Autodesk Inventor part; units mm, degrees
ref_plane "Work Plane1" through (29, 0, 0) normal (0, -1, 0) x (1, 0, 0)
ref_plane "YZ Plane" through (0, 0, 0) normal (1, 0, 0) x (0, 1, 0)
ref_plane "XZ Plane" through (0, 0, 0) normal (0, 1, 0) x (-1, 0, 0)
sketch "Sketch1" plane through (0, 0, 0) normal (0, 0, 1) x (1, 0, 0)
  line L0 (-0.0847, 0) -> (15.875, 0)
  line L1 (15.875, 0) -> (15.875, 2.0828)
  line L2 (15.875, 2.0828) -> (1.5902, 2.0828)
  line L3 (1.5902, 2.0828) -> (0.0001, 2.0828)
  line L4 (0.0001, 2.0828) -> (0, 2.0828)
  line L5 (0, 2.0828) -> (0, 3.9624)
  line L6 (0, 3.9624) -> (-2.2098, 3.9624)
  line L7 (-2.2098, 3.9624) -> (-2.2098, 1.3931)
  line L8 (-2.2098, 1.3931) -> (-0.889, 1.3931)
  line L9 (-0.889, 1.3931) -> (-0.0847, 0)
  line L10 (-21, 0) -> (56, 0)
  line L11 (0, -1.6) -> (0, 9.6)
  line L12 (1.5902, 2.0828) -> (0, 2.0828) construction
  dimension "d1" = 14.2848
  dimension "d2" = 1.5901
  dimension "d3" = 2.2098
  dimension "d4" = 1.3208
  dimension "d5" = 60
  dimension "d6" = 4.1656
  dimension "d7" = 4.1656
  dimension "d8" = 2.7863
  dimension "d9" = 7.9248
  dimension "d26" = 15.875
revolve "Body" add sketch "Sketch1" angle 360 about axis through (-0.0847, 0, 0) along (1, 0, 0)
sketch "Sketch2" plane through (-2.2098, 0, 0) normal (-1, 0, 0) x (0, 0, 1)
  circle A0 centre (0, 0) radius 1.3931
  line L0 (0, -6.4663) -> (0, 6.4663)
  line L1 (-6.4663, 0) -> (6.4663, 0)
  line L2 (1.3931, 0) -> (0.6966, -1.2065)
  line L3 (0.6966, -1.2065) -> (-0.6966, -1.2065)
  line L4 (-0.6966, -1.2065) -> (-1.3931, 0)
  line L5 (-1.3931, 0) -> (-0.6966, 1.2065)
  line L6 (-0.6966, 1.2065) -> (0.6966, 1.2065)
  line L7 (0.6966, 1.2065) -> (1.3931, 0)
extrude "Slot" add sketch "Sketch2" against normal up to next contours L7 A0 | A0 L2 | L6 L0 A0 | A0 L0 L3 | L0 L6 A0 | A0 L3 L0 | L4 A0 | A0 L5
fillet "Fillet1" radius 1.8288 1 edges at (-2.2098, -3.9624, 0)
thread "Thread"
chamfer "Chamfer1" distance 0.4204 distance2 0.4204 1 edges at (15.875, -2.0828, 0) measured on face at (15.875, -0.1898, 0.4203)
ref_plane "Work Plane1" through (29, 0, 0) normal (0, -1, 0) x (1, 0, 0)
fillet "Fillet2" radius 0.1 1 edges at (0.0001, -2.0828, 0)
equation "\"d1\" = GEL"
equation "\"d3\" = KOH"
equation "\"d4\" = INTI"
equation "\"d6\" = GD"
equation "\"d7\" = BDM"
equation "\"d8\" = 1.1547 * SW"
equation "\"d9\" = KOD"
equation "\"d26\" = NLG"
equation "\"d30\" = R"
equation "\"d17\" = RR"
equation "\"d13\" = GEL"
equation "\"d15\" = -0.5 * SPD + 0.5 * GD"
equation "\"d16\" = GUL"
equation "\"GD\" = NND"
equation "\"NLG\" = 15.875"
equation "\"GEL\" = 14.28476"
equation "\"KOD\" = 7.9248"
equation "\"KOH\" = 2.2098"
equation "\"INTI\" = 1.3208"
equation "\"GAL\" = 1.59004"
equation "\"GUL\" = 0.42037"
equation "\"BDM\" = NND"
equation "\"SW\" = 2.413"
equation "\"RR\" = 1.8288"
equation "\"SPD\" = 3.32486"
equation "\"R\" = 0.1"
equation "\"TOA\" = 30deg"
equation "\"GD1\" = SPD"
equation "\"THREADDIA\" = 4.1656"
equation "\"KOH1\" = 0.381"
equation "\"NND\" = 4.1656"
equation "\"E0\" = 2.78714"
properties part number "ANSI B18.3 - No. 8-36 - 5/8" material "Steel, Mild"
Build history of the part. All positions in model axes, mm. A direction names the side the tool comes from. Round coordinates to 2 decimals unless told otherwise and drop trailing zeros. Write each loop counter-clockwise with the first axis right and the second up, starting at its lowest first coordinate (ties: lowest second). Pieces come first, ordered by that corner, then holes.
1) Pin check, flat tips, straight feed: pin 1 (1.5 mm diameter, centred on y = 2, z = 1, fed in from -X); pin 2 (1 mm diameter, centred on x = 2, y = 1, fed in from -Z); pin 3 (2 mm diameter, centred on x = 12.5, z = 1.5, fed in from -Y); pin 4 (2 mm diameter, centred on x = 2, y = -1.5, fed in from +Z). Stop position of each tip, or through.
2) Mould opens along Z. For faces 1 (the conical face through (-0.14, -0.02, 0.09)), 2 (the flat face through (-2.21, -1, 1)), 3 (the cylindrical face through (7.67, 1.987, -0.626)) say: +Z half, -Z half, draft (parallel to the pull), parting line (faces both ways), or undercut.
3) Band-saw the part on A-A, the plane x = 3.25. List the corners of the cut face in (y, z).
4) Drill centre lines: probe 1 along Y at (x, z) = (10.25, 0); probe 2 along X at (y, z) = (-1, 2); probe 3 along X at (y, z) = (1.25, 2.5). Where is each one in solid material? Low to high.
5) 3-axis set-ups, long thin cutter, end or side, ignore diameter. For faces 4 (the cylindrical face through (-0.19, -0.52, -3.93)), 5 (the flat face through (-2, 1.206, 0)): which of +Z, -Z, +X, -X, +Y, -Y reach the whole face in a straight line?
Ans:
1. pin 1: stops at x = -2.21
1. pin 2: stops at z = -2.02
1. pin 3: stops at y = -2.02
1. pin 4: stops at z = 2.02
2. face 1: undercut
2. face 2: draft
2. face 3: parting line
3. outline: circle Ø4.17 at (0, 0)
4. probe 1: y = -2.08 to 2.08
4. probe 2: x = -2.21 to 0
4. probe 3: x = -2.09 to 0
5. face 4: +X, -X
5. face 5: -X
